Verification items for the finished model (mm, model axes). Face numbers are marked on the shaded views. Coordinates: 2 decimals unless noted, no trailing zeros. Order: outer loops, then holes, each group sorted by start corner. A loop starts at its lowest first (then second) coordinate and runs counter-clockwise, first axis right, second up.
Q1. Depth check by flat-ended pin: P1, Ø6, axis at x = 40.5, y = 8, coming from the +Z side; P2, Ø6, axis at x = 51.5, y = 16.5, coming from the -Z side. Enter the tip coordinate at first touch or a pass-through.
Q2. Cross-section at C-C, the plane x = 90.5. Record the boundary of the cut face in (y, z).
Q3. Cross-section at D-D, the plane z = 210.5. Record the boundary of the cut face in (x, y).
Q4. Cross-section at B-B, the plane z = 28. Record the boundary of the cut face in (x, y), and give its area (3 significant figures).
Q5. Draft check along X on the marked faces 1, 2 and 3. Enter one of: pulls with the +X half, pulls with the -X half, needs draft (parallel to the pull), parting line crosses it, or undercut.
Q6. Cross-section at A-A, the plane y = 7. Record the boundary of the cut face in (x, z), and give its area (3 significant figures).
Q7. Thickness scan on line 1 (X direction, y = 2.5, z = 204.5); line 2 (Y direction, x = 139, z = 125); line 3 (Z direction, x = 39, y = 32.5). Record the ranges inside material, lowest first.
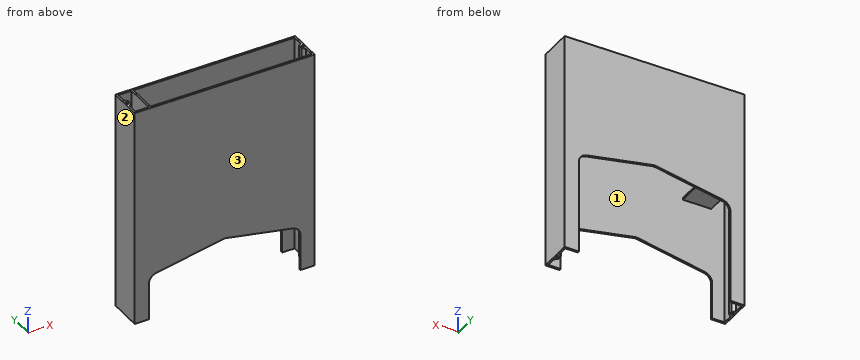
from build123d import *

# Parameters (mm, degrees)
F0_W     = 190
F0_H     = 35
F0_R     = 1.5
F1_DEPTH = 232
F2_W     = 2
F2_H     = 110
F2_H_2   = 2
F2_W_2   = 28
F3_DEPTH = 33
F4_W     = 160
F4_H     = 107
F5_DEPTH = 5
F6_W     = 160
F6_H     = 47
F7_DEPTH = 5
F8_R     = 10


with BuildPart() as f1:
    # F0 (on Top) → F1 (new body)
    with BuildSketch(Plane.XY):
        with Locations((95, 17.5)):
            Rectangle(F0_W, F0_H)
        with Locations((2, 17.5)):
            Circle(F0_R, mode=Mode.SUBTRACT)
        Polygon((188, 2), (2, 2), (2, 12.3786796564), (5, 15.3786796564), (5, 19.6213203436), (2, 22.6213203436), (2, 33), (188, 33), (188, 22.6213203436), (185, 19.6213203436), (185, 15.3786796564), (188, 12.3786796564), align=None, mode=Mode.SUBTRACT)
        with Locations((188, 17.5)):
            Circle(F0_R, mode=Mode.SUBTRACT)
    extrude(amount=F1_DEPTH)

    # F2 (on face) → F3 (join)
    with BuildSketch(Plane.XZ):
        with Locations((17, 177)):
            Rectangle(F2_W, F2_H)
        with Locations((17, 121)):
            Rectangle(F2_W, F2_H_2)
        with Locations((32, 121)):
            Rectangle(F2_W_2, F2_H_2)
    extrude(amount=-F3_DEPTH)

    # F4 (on face) → F5 (cut)
    with BuildSketch(Plane(origin=(0, 35, 0), x_dir=(-1, 0, 0), z_dir=(0, 1, 0))):
        with Locations((-95, 53.5)):
            Rectangle(F4_W, F4_H)
        Polygon((-175, 107), (-15, 107), (-95, 122), align=None)
    extrude(amount=-F5_DEPTH, mode=Mode.SUBTRACT)

    # F6 (on face) → F7 (cut)
    with BuildSketch(Plane.XZ):
        Polygon((95, 62), (15, 47), (175, 47), align=None)
        with Locations((95, 23.5)):
            Rectangle(F6_W, F6_H)
    extrude(amount=-F7_DEPTH, mode=Mode.SUBTRACT)

    # F8
    f8_edges = [f1.edges().sort_by_distance(p)[0] for p in [
        (175, 1, 47),
        (175, 34, 107),
        (15, 34, 107),
        (15, 1, 47),
        (95, 34, 122),
        (95, 1, 62),
    ]]
    fillet(f8_edges, radius=F8_R)


solid = f1.part
Check values:
1. P1: stops at z = 122
1. P2: passes through
2. outline: (0, 61.16) - (2, 61.16) - (2, 232) - (0, 232) - close; (33, 121.16) - (35, 121.16) - (35, 232) - (33, 232) - close
3. outline: (0, 0) - (190, 0) - (190, 35) - (0, 35) - close; hole circle Ø3 at (2, 17.5); hole (2, 2) - (16, 2) - (16, 33) - (2, 33) - (2, 22.62) - (5, 19.62) - (5, 15.38) - (2, 12.38) - close; hole (18, 2) - (188, 2) - (188, 12.38) - (185, 15.38) - (185, 19.62) - (188, 22.62) - (188, 33) - (18, 33) - close; hole circle Ø3 at (188, 17.5)
4. outline: (0, 0) - (15, 0) - (15, 2) - (2, 2) - (2, 12.38) - (5, 15.38) - (5, 19.62) - (2, 22.62) - (2, 33) - (15, 33) - (15, 35) - (0, 35) - close; (175, 0) - (190, 0) - (190, 35) - (175, 35) - (175, 33) - (188, 33) - (188, 22.62) - (185, 19.62) - (185, 15.38) - (188, 12.38) - (188, 2) - (175, 2) - close; hole circle Ø3 at (2, 17.5); hole circle Ø3 at (188, 17.5)
4. area: 273 mm2
5. face 1: undercut
5. face 2: pulls with the -X half
5. face 3: needs draft
6. outline: (0, 0) - (2, 0) - (2, 232) - (0, 232) - close; (16, 120) - (46, 120) - (46, 122) - (18, 122) - (18, 232) - (16, 232) - close; (188, 0) - (190, 0) - (190, 232) - (188, 232) - close
6. area: 1,210 mm2
7. line 1: x = 0 to 2, 16 to 18, 188 to 190
7. line 2: y = 0 to 2, 33 to 35
7. line 3: z = 120 to 122
